Job drawing, mm, ordinate dimensions from the low corner. One solid piece. Round coordinates to 2 decimals unless told otherwise and drop trailing zeros. Loops run counter-clockwise (first coordinate to the right, second up) from the corner with the lowest first, then second, coordinate; pieces in that order, holes last. Notation, with made-up numbers: M 71,39.25 L 102,39.25 A6 cw 102,46.25 Z; hole C 5.5,-25 d7. An arc over 180 degrees is marked long. Put each result on its own line as item: value. Start each with the question number.
1) Pull direction Z, two halves, no side cores. Call the marked faces 1, 2, 3 and 4: +Z half, -Z half, draft (parallel to the pull), parting line (faces both ways), or undercut.
2) Slice it at D-D on z = 5.5. Give the cut face in (x, y).
3) Probe line 1 along Y through (x, z) = (11, 5); line 2 along Y through (x, z) = (18, 0.5); line 3 along X through (y, z) = (12, 5.5). List the from-to ranges inside material, lowest first.
4) Drop flat-ended pins along their axis: pin 1 Ø1.5 at (y, z) = (20.5, 6) entering from -X; pin 2 Ø1.5 at (y, z) = (18, 3) entering from -X; pin 3 Ø2 at (y, z) = (18.5, 2) entering from +X; pin 4 Ø18 at (x, y) = (16, 16) entering from +Z. Give the stop position or say it passes through.
5) Slice it at C-C on z = 0.5. Give the cut face in (x, y).
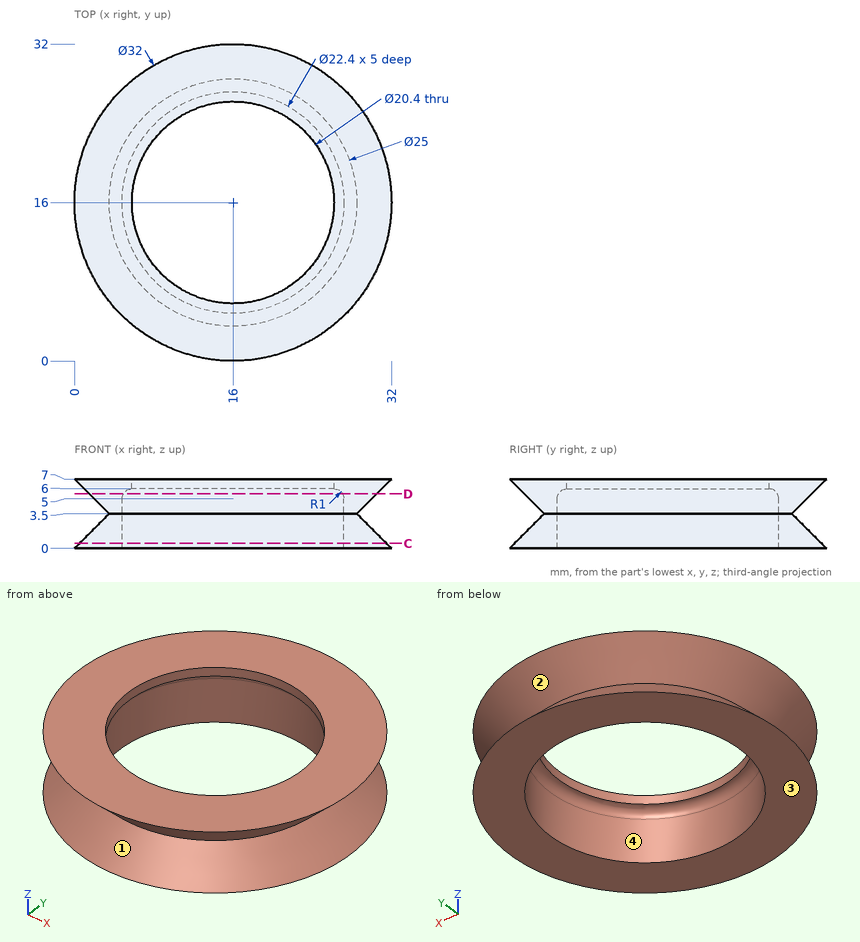
Recorded:
1. face 1: undercut
1. face 2: undercut
1. face 3: -Z half
1. face 4: draft
2. outline: C 16,16 d29; hole C 16,16 d22.13
3. line 1: y = 2.92 to 5.98, 26.02 to 29.08
3. line 2: y = 0.63 to 4.98, 27.02 to 31.37
3. line 3: x = 2.06 to 5.68, 26.32 to 29.94
4. pin 1: stops at x = 0.88
4. pin 2: stops at x = 2.39
4. pin 3: stops at x = 30.8
4. pin 4: passes through
5. outline: C 16,16 d31; hole C 16,16 d22.4
